Design review of the part shown in the three views and the two pictorial views. Dimensions are in mm from the part's minimum x, y and z. A direction names the side the tool comes from. Coordinates: 2 decimals unless noted, no trailing zeros. Order: outer loops, then holes, each group sorted by start corner. A loop starts at its lowest first (then second) coordinate and runs counter-clockwise, first axis right, second up. Notation, with made-up numbers: (55, 19) - (103, 19) arc R17 ccw to (103, 27) - close; hole circle Ø8 at (-17.5, 69.5). An arc over 180 degrees is marked (long way). One line per item, written item: value. Start each with the question number.
(1) Mouldability with a two-part tool opening along Y and no side actions: class the marked faces 1, 2 and 3 as released by +Y, released by -Y, zero draft, split by the parting line, or undercut.
(2) Consider section A-A on y = 2.5. Write out the cut boundary in (x, z), then the cut area to 3 significant figures.
(3) Clearance check with flat-ended pins moving along their axes: pin 1 (0.6 mm diameter, centred on x = 1.5, z = 0.5, fed in from +Y) (3 decimals); pin 2 (1.4 mm diameter, centred on x = 13.45, y = 16.955, fed in from +Z). State where each tip first meets the part, or that it passes through.
(4) Consider section C-C on z = 1.2. Write out the cut boundary in (x, y) (3 decimals).
(5) Consider section B-B on x = 13.45. Write out the cut boundary in (y, z) (3 decimals), then the cut area to 3 significant figures.
(6) For the marked faces 4, 5 and 6, list the 3-axis set-ups (+Z, -Z, +X, -X, +Y, -Y) from which the entire face can be reached by the end or side of a thin tool; tool diameter is ignored.
(7) Consider section D-D on y = 16.5. Write out the cut boundary in (x, z), then the cut area to 3 significant figures.
(8) To check wall thickness, follow line 1 along Y through (x, z) = (3.75, 0.2) (3 decimals); line 2 along X through (y, z) = (2.5, 0.6); line 3 along Y through (x, z) = (2.75, 0.8) (3 decimals). State the ranges of each line that lie inside material, in increasing order.
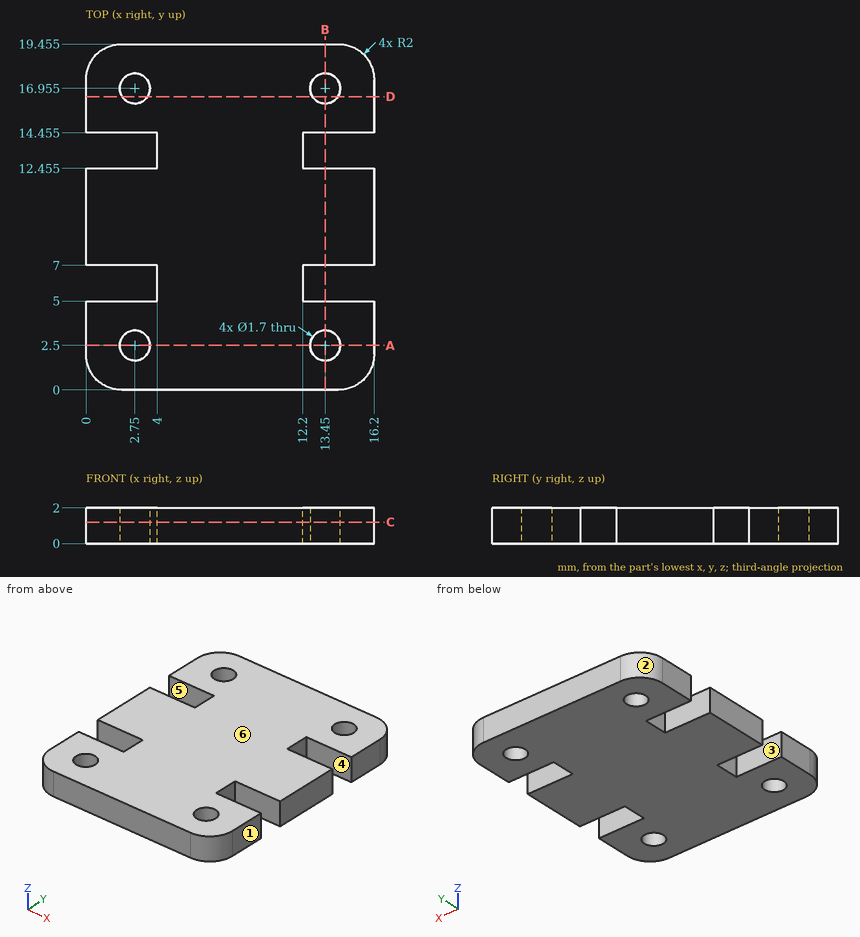
Geometry check:
1. face 1: zero draft
1. face 2: released by +Y
1. face 3: undercut
2. outline: (0, 0) - (1.9, 0) - (1.9, 2) - (0, 2) - close; (3.6, 0) - (12.6, 0) - (12.6, 2) - (3.6, 2) - close; (14.3, 0) - (16.2, 0) - (16.2, 2) - (14.3, 2) - close
2. area: 25.6 mm^2
3. pin 1: stops at y = 19.445
3. pin 2: passes through
4. outline: (0, 2) arc R2 ccw to (2, 0) - (14.2, 0) arc R2 ccw to (16.2, 2) - (16.2, 5) - (12.2, 5) - (12.2, 7) - (16.2, 7) - (16.2, 12.455) - (12.2, 12.455) - (12.2, 14.455) - (16.2, 14.455) - (16.2, 17.455) arc R2 ccw to (14.2, 19.455) - (2, 19.455) arc R2 ccw to (0, 17.455) - (0, 14.455) - (4, 14.455) - (4, 12.455) - (0, 12.455) - (0, 7) - (4, 7) - (4, 5) - (0, 5) - close; hole circle Ø1.7 at (2.75, 2.5); hole circle Ø1.7 at (2.75, 16.955); hole circle Ø1.7 at (13.45, 2.5); hole circle Ø1.7 at (13.45, 16.955)
5. outline: (0, 0) - (1.65, 0) - (1.65, 2) - (0, 2) - close; (3.35, 0) - (5, 0) - (5, 2) - (3.35, 2) - close; (7, 0) - (12.455, 0) - (12.455, 2) - (7, 2) - close; (14.455, 0) - (16.105, 0) - (16.105, 2) - (14.455, 2) - close; (17.805, 0) - (19.455, 0) - (19.455, 2) - (17.805, 2) - close
5. area: 24.1 mm^2
6. face 4: +Z, -Z, +X
6. face 5: +Z, -Z, -X
6. face 6: +Z, +X, -X, +Y, -Y
7. outline: (0, 0) - (2.03, 0) - (2.03, 2) - (0, 2) - close; (3.47, 0) - (12.73, 0) - (12.73, 2) - (3.47, 2) - close; (14.17, 0) - (16.2, 0) - (16.2, 2) - (14.17, 2) - close
7. area: 26.7 mm^2
8. line 1: y = 0 to 5, 7 to 12.455, 14.455 to 19.455
8. line 2: x = 0 to 1.9, 3.6 to 12.6, 14.3 to 16.2
8. line 3: y = 0 to 1.65, 3.35 to 5, 7 to 12.455, 14.455 to 16.105, 17.805 to 19.455
